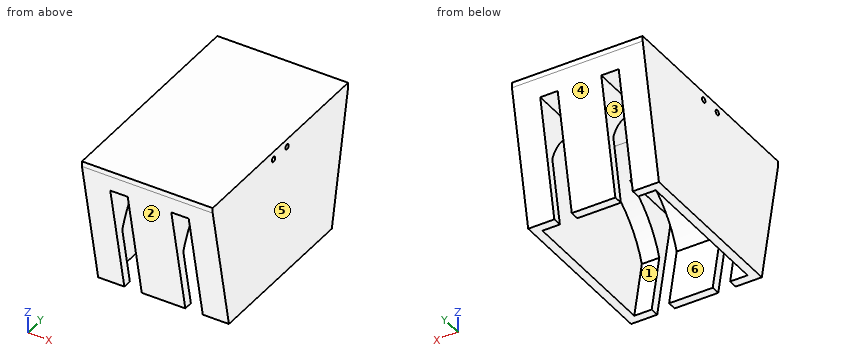
from build123d import *

# Parameters (mm, degrees)
BOSS_EXTRUDE1_DEPTH     = 37.5
SHELL1_T                = -5
BOSS_EXTRUDE4_DEPTH     = 65
CUT_EXTRUDE4_DEPTH      = 82.967981554
CUT_EXTRUDE4_DEPTH_BACK = 82.967981554
SKETCH11_W              = 10
SKETCH11_H              = 65
SKETCH13_W              = 75
SKETCH13_H              = 125
BOSS_EXTRUDE5_DEPTH     = 3
SKETCH12_R              = 1.5
CUT_EXTRUDE5_DEPTH      = 106.695316831


with BuildPart() as part:
    # Sketch1 → Boss-Extrude1 (new, symmetric)
    with BuildSketch(Plane(origin=(0, 0, 0), x_dir=(0, 0, -1), z_dir=(1, 0, 0))):
        Polygon((-37.5, 32.5), (-37.5, -52.5), (-37.5, -62.5), (37.5, -47.5), (37.5, -37.5), (37.5, -32.5), (37.5, 32.5), (37.5, 47.5), (-37.5, 62.5), (-37.5, 47.5), align=None)
    extrude(amount=BOSS_EXTRUDE1_DEPTH, both=True)

    # Shell1
    shell1_openings = [part.faces().sort_by_distance(p)[0] for p in [
        (0, 0, -37.5),
    ]]
    offset(amount=SHELL1_T, openings=shell1_openings, kind=Kind.INTERSECTION)

    # Sketch10 → Boss-Extrude4 (add)
    with BuildSketch(Plane.ZY.offset(-32.5)):
        with BuildLine():
            Line((-2.5, -49.400980486), (32.5, -56.400980486))
            Line((32.5, -56.400980486), (32.5, 0))
            ThreePointArc((32.5, 0), (22.863250205, -30.271508358), (-2.5, -49.400980486))
        make_face()
        with BuildLine():
            ThreePointArc((-2.5, 49.400980486), (22.863250205, 30.271508358), (32.5, 0))
            Line((32.5, 0), (32.5, 56.400980486))
            Line((32.5, 56.400980486), (-2.5, 49.400980486))
        make_face()
    extrude(amount=BOSS_EXTRUDE4_DEPTH)

    # Sketch11 → Cut-Extrude4 (cut, two sides: drawn at the far end of the back side and taken through both)
    with BuildSketch(Plane(origin=(0, 0, 0), x_dir=(1, 0, 0), z_dir=(0, 1, 0)).offset(-CUT_EXTRUDE4_DEPTH_BACK)):
        with Locations((-17.5, 5)):
            Rectangle(SKETCH11_W, SKETCH11_H)
        with Locations((17.5, 5)):
            Rectangle(SKETCH11_W, SKETCH11_H)
    extrude(amount=CUT_EXTRUDE4_DEPTH + CUT_EXTRUDE4_DEPTH_BACK, mode=Mode.SUBTRACT)

    # Sketch13 → Boss-Extrude5 (add)
    with BuildSketch(Plane.XY.offset(37.5)):
        Rectangle(SKETCH13_W, SKETCH13_H)
    extrude(amount=BOSS_EXTRUDE5_DEPTH)

    # Sketch12 → Cut-Extrude5 (cut, through all)
    with BuildSketch(Plane(origin=(37.5, 0, 0), x_dir=(0, 0, -1), z_dir=(1, 0, 0))):
        with Locations((-36, 6.15)):
            Circle(SKETCH12_R)
        with Locations(Location((-36, -6.35, 0), (0, 0, 180))):
            Circle(SKETCH12_R)
    extrude(amount=-CUT_EXTRUDE5_DEPTH, mode=Mode.SUBTRACT)


solid = part.part
Build history of the part. All positions in model axes, mm. Face numbers are marked on the shaded views. A direction names the side the tool comes from. Give positions to 0.01 mm unless a question says otherwise; leave off trailing zeros. Write each loop counter-clockwise with the first axis right and the second up, starting at its lowest first coordinate (ties: lowest second). Pieces come first, ordered by that corner, then holes. Notation, with made-up numbers: (44.25, -33.5) - (70.25, -33.5) arc R4 ccw to (70.25, -29.5) - close; hole circle Ø5 at (38, -6). An arc over 180 degrees is marked (long way). Use one line per item in the form item = value. Start each with the question number.
1. Two-plate mould, pull along Z, no slides. Class the marked faces 4, 5 and 6: released by +Z, released by -Z, zero draft, split by the parting line, or undercut.
2. Probe line 1 (X direction, y = 45, z = 7); line 2 (X direction, y = -26.5, z = 9); line 3 (Y direction, x = -1, z = 36). List the from-to ranges inside material, lowest first. Write a range as [from, to].
3. 3-axis set-ups, long thin cutter, end or side, ignore diameter. For the marked faces 1, 2 and 3: which of +Z, -Z, +X, -X, +Y, -Y reach the whole face in a straight line?
4. Band-saw the part on D-D on z = -14. Write the cut outline in (x, y), plus the area to 3 significant figures.
5. Drop flat-ended pins along their axis: pin 1 Ø4 at (x, z) = (7, 17.5) entering from -Y; pin 2 Ø1.8 at (y, z) = (-6.35, 36) entering from +X; pin 3 Ø3 at (x, y) = (-15.5, 41) entering from -Z; pin 4 Ø5 at (y, z) = (6.15, 36) entering from -X. Give the stop position or say it passes through.
6. Band-saw the part on C-C on y = -52.5. Write the cut outline in (x, z), plus the area to 4 significant figures.
7. Band-saw the part on A-A on z = 36. Write the cut outline in (x, y), plus the area to 3 significant figures.
8. Band-saw the part on B-B on x = -25.5. Write the cut outline in (y, z), plus the area to 3 significant figures.
Conclusion:
q1.face_4 = released by -Z
q1.face_5 = zero draft
q1.face_6 = undercut
q2.line_1 = [-37.5, -22.5], [-12.5, 12.5], [22.5, 37.5]
q2.line_2 = [-37.5, -32.5], [32.5, 37.5]
q2.line_3 = [-62.2, -7.85], [-4.85, 4.65], [7.65, 62.2]
q3.face_1 = none
q3.face_2 = -Z, +X, -X, -Y
q3.face_3 = -Z, +Y, -Y
q4.outline = (-37.5, -52.2) - (-22.5, -52.2) - (-22.5, -47.1) - (-32.5, -47.1) - (-32.5, 47.1) - (-22.5, 47.1) - (-22.5, 52.2) - (-37.5, 52.2) - close; (-12.5, -52.2) - (12.5, -52.2) - (12.5, -47.1) - (-12.5, -47.1) - close; (-12.5, 47.1) - (12.5, 47.1) - (12.5, 52.2) - (-12.5, 52.2) - close; (22.5, -52.2) - (37.5, -52.2) - (37.5, 52.2) - (22.5, 52.2) - (22.5, 47.1) - (32.5, 47.1) - (32.5, -47.1) - (22.5, -47.1) - close
q4.area = 1,500 mm²
q5.pin_1 = -58.9
q5.pin_2 = through
q5.pin_3 = 27.5
q5.pin_4 = -37.5
q6.outline = (-37.5, -12.5) - (-22.5, -12.5) - (-22.5, 27.5) - (-12.5, 27.5) - (-12.5, -12.5) - (12.5, -12.5) - (12.5, 27.5) - (22.5, 27.5) - (22.5, -12.5) - (37.5, -12.5) - (37.5, 40.5) - (-37.5, 40.5) - close
q6.area = 3,175 mm²
q7.outline = (-37.5, -62.2) - (37.5, -62.2) - (37.5, -7.85) - (-37.5, -7.85) - close; (-37.5, -4.85) - (37.5, -4.85) - (37.5, 4.65) - (-37.5, 4.65) - close; (-37.5, 7.65) - (37.5, 7.65) - (37.5, 62.2) - (-37.5, 62.2) - close
q7.area = 8,880 mm²
q8.outline = (-62.5, 37.5) - (-47.5, -37.5) - (-42.4, -37.5) - (-49.4, -2.5) arc R52.36 cw to (49.4, -2.5) - (42.4, -37.5) - (47.5, -37.5) - (62.5, 37.5) - (62.5, 40.5) - (-62.5, 40.5) - close; hole circle Ø3 at (-6.35, 36); hole circle Ø3 at (6.15, 36)
q8.area = 2,880 mm²
